Read the model definition and answer for the solid it produces. Units are mm, in the model's axes. Give positions to 0.01 mm unless a question says otherwise; leave off trailing zeros. Order: outer loops, then holes, each group sorted by start corner. A loop starts at its lowest first (then second) coordinate and runs counter-clockwise, first axis right, second up. Notation, with made-up numbers: (-36, 31) - (-22, 31) arc R21 cw to (-22, 51) - close; hole circle Ø10 at (76.25, 11.25). An arc over 180 degrees is marked (long way). Answer as CSV lines item,"result". Start each with the question number.
from build123d import *

# Parameters (mm, degrees)
SKETCH_1_W          = 9
SKETCH_1_H          = 6.5
EXTRUDE_1_DEPTH     = 100
SKETCH_2_R          = 1.750000006
CUT_EXTRUDE_1_DEPTH = 90.614230596
SKETCH_3_R          = 3.000000006
CUT_EXTRUDE_2_DEPTH = 3.5


with BuildPart() as part:
    # 草图1 → 凸台-拉伸1 (new body)
    with BuildSketch(Plane.XY.offset(-89.264832522)):
        Rectangle(SKETCH_1_W, SKETCH_1_H)
    extrude(amount=EXTRUDE_1_DEPTH)

    # 草图2 → 切除-拉伸1 (cut, through all)
    with BuildSketch(Plane(origin=(0, 3.25, 0), x_dir=(1, 0, 0), z_dir=(0, 1, 0))):
        with Locations(Location((0, 81.764832522, 0), (0, 0, 270))):
            Circle(SKETCH_2_R)
        with Locations(Location((0, 61.764832522, 0), (0, 0, 270))):
            Circle(SKETCH_2_R)
        with Locations(Location((0, 41.764832522, 0), (0, 0, 270))):
            Circle(SKETCH_2_R)
        with Locations(Location((0, 21.764832522, 0), (0, 0, 270))):
            Circle(SKETCH_2_R)
        with Locations(Location((0, 1.764832522, 0), (0, 0, 270))):
            Circle(SKETCH_2_R)
        with Locations((0, -18.235167478)):
            Circle(SKETCH_2_R)
        with Locations((0, -38.235167478)):
            Circle(SKETCH_2_R)
        with Locations((0, -58.235167478)):
            Circle(SKETCH_2_R)
        with Locations((0, -78.235167478)):
            Circle(SKETCH_2_R)
        with Locations((0, -98.235167478)):
            Circle(SKETCH_2_R)
        with Locations((0, -118.235167478)):
            Circle(SKETCH_2_R)
        with Locations((0, -138.235167478)):
            Circle(SKETCH_2_R)
        with Locations((0, -158.235167478)):
            Circle(SKETCH_2_R)
        with Locations((0, -178.235167478)):
            Circle(SKETCH_2_R)
        with Locations((0, -198.235167478)):
            Circle(SKETCH_2_R)
        with Locations((0, -218.235167478)):
            Circle(SKETCH_2_R)
        with Locations((0, -238.235167478)):
            Circle(SKETCH_2_R)
        with Locations((0, -258.235167478)):
            Circle(SKETCH_2_R)
        with Locations((0, -278.235167478)):
            Circle(SKETCH_2_R)
        with Locations((0, -298.235167478)):
            Circle(SKETCH_2_R)
        with Locations((0, -318.235167478)):
            Circle(SKETCH_2_R)
        with Locations((0, -338.235167478)):
            Circle(SKETCH_2_R)
        with Locations((0, -358.235167478)):
            Circle(SKETCH_2_R)
        with Locations((0, -378.235167478)):
            Circle(SKETCH_2_R)
        with Locations((0, -398.235167478)):
            Circle(SKETCH_2_R)
        with Locations((0, -418.235167478)):
            Circle(SKETCH_2_R)
        with Locations((0, -438.235167478)):
            Circle(SKETCH_2_R)
        with Locations((0, -458.235167478)):
            Circle(SKETCH_2_R)
        with Locations((0, -478.235167478)):
            Circle(SKETCH_2_R)
        with Locations((0, -498.235167478)):
            Circle(SKETCH_2_R)
        with Locations((0, -518.235167478)):
            Circle(SKETCH_2_R)
        with Locations((0, -538.235167478)):
            Circle(SKETCH_2_R)
        with Locations((0, -558.235167478)):
            Circle(SKETCH_2_R)
        with Locations((0, -578.235167478)):
            Circle(SKETCH_2_R)
        with Locations((0, -598.235167478)):
            Circle(SKETCH_2_R)
        with Locations((0, -618.235167478)):
            Circle(SKETCH_2_R)
        with Locations((0, -638.235167478)):
            Circle(SKETCH_2_R)
        with Locations((0, -658.235167478)):
            Circle(SKETCH_2_R)
        with Locations((0, -678.235167478)):
            Circle(SKETCH_2_R)
        with Locations((0, -698.235167478)):
            Circle(SKETCH_2_R)
        with Locations((0, -718.235167478)):
            Circle(SKETCH_2_R)
        with Locations((0, -738.235167478)):
            Circle(SKETCH_2_R)
        with Locations((0, -758.235167478)):
            Circle(SKETCH_2_R)
        with Locations((0, -778.235167478)):
            Circle(SKETCH_2_R)
        with Locations((0, -798.235167478)):
            Circle(SKETCH_2_R)
        with Locations((0, -818.235167478)):
            Circle(SKETCH_2_R)
        with Locations((0, -838.235167478)):
            Circle(SKETCH_2_R)
        with Locations((0, -858.235167478)):
            Circle(SKETCH_2_R)
        with Locations((0, -878.235167478)):
            Circle(SKETCH_2_R)
        with Locations((0, -898.235167478)):
            Circle(SKETCH_2_R)
        with Locations((0, -918.235167478)):
            Circle(SKETCH_2_R)
        with Locations((0, -938.235167478)):
            Circle(SKETCH_2_R)
        with Locations((0, -958.235167478)):
            Circle(SKETCH_2_R)
        with Locations((0, -978.235167478)):
            Circle(SKETCH_2_R)
        with Locations((0, -998.235167478)):
            Circle(SKETCH_2_R)
        with Locations((0, -1018.235167478)):
            Circle(SKETCH_2_R)
        with Locations((0, -1038.235167478)):
            Circle(SKETCH_2_R)
        with Locations((0, -1058.235167478)):
            Circle(SKETCH_2_R)
        with Locations((0, -1078.235167478)):
            Circle(SKETCH_2_R)
        with Locations((0, -1098.235167478)):
            Circle(SKETCH_2_R)
    extrude(amount=-CUT_EXTRUDE_1_DEPTH, mode=Mode.SUBTRACT)

    # 草图3 → 切除-拉伸2 (cut)
    with BuildSketch(Plane(origin=(0, 3.25, 0), x_dir=(1, 0, 0), z_dir=(0, 1, 0))):
        with Locations(Location((0, 81.764832522, 0), (0, 0, 270))):
            Circle(SKETCH_3_R)
        with Locations(Location((0, 61.764832522, 0), (0, 0, 270))):
            Circle(SKETCH_3_R)
        with Locations(Location((0, 41.764832522, 0), (0, 0, 270))):
            Circle(SKETCH_3_R)
        with Locations(Location((0, 21.764832522, 0), (0, 0, 270))):
            Circle(SKETCH_3_R)
        with Locations(Location((0, 1.764832522, 0), (0, 0, 270))):
            Circle(SKETCH_3_R)
        with Locations((0, -18.235167478)):
            Circle(SKETCH_3_R)
        with Locations((0, -38.235167478)):
            Circle(SKETCH_3_R)
        with Locations((0, -58.235167478)):
            Circle(SKETCH_3_R)
        with Locations((0, -78.235167478)):
            Circle(SKETCH_3_R)
        with Locations((0, -98.235167478)):
            Circle(SKETCH_3_R)
        with Locations((0, -118.235167478)):
            Circle(SKETCH_3_R)
        with Locations((0, -138.235167478)):
            Circle(SKETCH_3_R)
        with Locations((0, -158.235167478)):
            Circle(SKETCH_3_R)
        with Locations((0, -178.235167478)):
            Circle(SKETCH_3_R)
        with Locations((0, -198.235167478)):
            Circle(SKETCH_3_R)
        with Locations((0, -218.235167478)):
            Circle(SKETCH_3_R)
        with Locations((0, -238.235167478)):
            Circle(SKETCH_3_R)
        with Locations((0, -258.235167478)):
            Circle(SKETCH_3_R)
        with Locations((0, -278.235167478)):
            Circle(SKETCH_3_R)
        with Locations((0, -298.235167478)):
            Circle(SKETCH_3_R)
        with Locations((0, -318.235167478)):
            Circle(SKETCH_3_R)
        with Locations((0, -338.235167478)):
            Circle(SKETCH_3_R)
        with Locations((0, -358.235167478)):
            Circle(SKETCH_3_R)
        with Locations((0, -378.235167478)):
            Circle(SKETCH_3_R)
        with Locations((0, -398.235167478)):
            Circle(SKETCH_3_R)
        with Locations((0, -418.235167478)):
            Circle(SKETCH_3_R)
        with Locations((0, -438.235167478)):
            Circle(SKETCH_3_R)
        with Locations((0, -458.235167478)):
            Circle(SKETCH_3_R)
        with Locations((0, -478.235167478)):
            Circle(SKETCH_3_R)
        with Locations((0, -498.235167478)):
            Circle(SKETCH_3_R)
        with Locations((0, -518.235167478)):
            Circle(SKETCH_3_R)
        with Locations((0, -538.235167478)):
            Circle(SKETCH_3_R)
        with Locations((0, -558.235167478)):
            Circle(SKETCH_3_R)
        with Locations((0, -578.235167478)):
            Circle(SKETCH_3_R)
        with Locations((0, -598.235167478)):
            Circle(SKETCH_3_R)
        with Locations((0, -618.235167478)):
            Circle(SKETCH_3_R)
        with Locations((0, -638.235167478)):
            Circle(SKETCH_3_R)
        with Locations((0, -658.235167478)):
            Circle(SKETCH_3_R)
        with Locations((0, -678.235167478)):
            Circle(SKETCH_3_R)
        with Locations((0, -698.235167478)):
            Circle(SKETCH_3_R)
        with Locations((0, -718.235167478)):
            Circle(SKETCH_3_R)
        with Locations((0, -738.235167478)):
            Circle(SKETCH_3_R)
        with Locations((0, -758.235167478)):
            Circle(SKETCH_3_R)
        with Locations((0, -778.235167478)):
            Circle(SKETCH_3_R)
        with Locations((0, -798.235167478)):
            Circle(SKETCH_3_R)
        with Locations((0, -818.235167478)):
            Circle(SKETCH_3_R)
        with Locations((0, -838.235167478)):
            Circle(SKETCH_3_R)
        with Locations((0, -858.235167478)):
            Circle(SKETCH_3_R)
        with Locations((0, -878.235167478)):
            Circle(SKETCH_3_R)
        with Locations((0, -898.235167478)):
            Circle(SKETCH_3_R)
        with Locations((0, -918.235167478)):
            Circle(SKETCH_3_R)
        with Locations((0, -938.235167478)):
            Circle(SKETCH_3_R)
        with Locations((0, -958.235167478)):
            Circle(SKETCH_3_R)
        with Locations((0, -978.235167478)):
            Circle(SKETCH_3_R)
        with Locations((0, -998.235167478)):
            Circle(SKETCH_3_R)
        with Locations((0, -1018.235167478)):
            Circle(SKETCH_3_R)
        with Locations((0, -1038.235167478)):
            Circle(SKETCH_3_R)
        with Locations((0, -1058.235167478)):
            Circle(SKETCH_3_R)
        with Locations((0, -1078.235167478)):
            Circle(SKETCH_3_R)
        with Locations((0, -1098.235167478)):
            Circle(SKETCH_3_R)
    extrude(amount=-CUT_EXTRUDE_2_DEPTH, mode=Mode.SUBTRACT)


solid = part.part
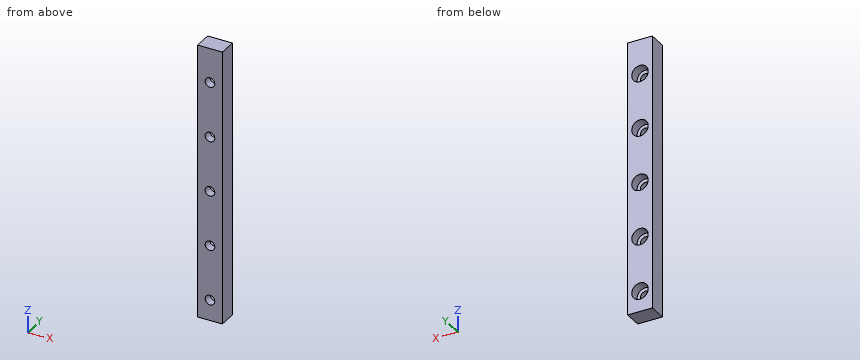
(1) Straight lines are drawn through the part: line 1 (Z direction, x = -0.25, y = -1); line 2 (X direction, y = 0, z = -22); line 3 (X direction, y = -2.75, z = -82). For each, find the intervals that lie inside material, in ascending order. Write a range as [from, to].
(2) Section B-B, the plane x = 0 is taken. State how many separate pieces and enclosed holes the cut face has, and give its area (4 significant figures).
(3) Section A-A, the plane y = -2.25 is taken. Write down the section's boundary in (x, z), and give its area (3 significant figures).
(4) Flat-ended cylindrical pins translate along their axes: pin 1 Ø5 at (x, z) = (1.5, -41) entering from +Y; pin 2 Ø3 at (x, z) = (0.5, -20.5) entering from +Y. Find the tip coordinate at first contact, or state that the pin passes through.
(5) Section C-C, the plane y = 1.75 is taken. Write down the section's boundary in (x, z).
Checks:
1,line 1,"z = [-89.26, -83.5], [-80.03, -63.5], [-60.03, -43.5], [-40.03, -23.5], [-20.03, -3.5], [-0.03, 10.74]"
1,line 2,"x = [-4.5, -2.99], [2.99, 4.5]"
1,line 3,"x = [-4.5, -1.73], [1.73, 4.5]"
2,separate pieces,"6"
2,enclosed holes,"0"
2,area,"492.5 mm²"
3,outline,"(-4.5, -89.26) - (4.5, -89.26) - (4.5, 10.74) - (-4.5, 10.74) - close; hole circle Ø3.5 at (0, -81.76); hole circle Ø3.5 at (0, -61.76); hole circle Ø3.5 at (0, -41.76); hole circle Ø3.5 at (0, -21.76); hole circle Ø3.5 at (0, -1.76)"
3,area,"852 mm²"
4,pin 1,"stops at y = 3.25"
4,pin 2,"stops at y = -0.25"
5,outline,"(-4.5, -89.26) - (4.5, -89.26) - (4.5, 10.74) - (-4.5, 10.74) - close; hole circle Ø6 at (0, -81.76); hole circle Ø6 at (0, -61.76); hole circle Ø6 at (0, -41.76); hole circle Ø6 at (0, -21.76); hole circle Ø6 at (0, -1.76)"
